Read the model definition and answer for the solid it produces. Units are mm, in the model's axes. A direction names the side the tool comes from. Coordinates: 2 decimals unless noted, no trailing zeros. Order: outer loops, then holes, each group sorted by start corner. A loop starts at its lowest first (then second) coordinate and runs counter-clockwise, first axis right, second up. Notation, with made-up numbers: M 63,69 L 106,69 A21 ccw 106,104 Z; hole C 9,69 d8. An arc over 180 degrees is marked long. One line per question, with ' | ' between items. Start each with the question number.
1) Consider probe 1 along X at (y, z) = (18.7, 40); probe 2 along Z at (x, y) = (-51.5, -15); probe 3 along Y at (x, z) = (65, 32). Determine where each line is inside the solid, lowest interval first.
2) Find section D-D, the plane z = 26. Write down the section's boundary in (x, y).
3) Find section A-A, the plane y = 0. Write down the section's boundary in (x, z), plus the area to 3 significant figures.
4) Given P1, Ø17.5, axis at x = -3.5, y = 2.5, coming from the +Z side; P2, Ø5, axis at y = 0.5, z = 6.5, coming from the -X side; P3, Ø5, axis at x = 53, z = 11, coming from the -Y side, each flat-ended and moving along its own axis, determine where each tip first touches the part or whether it passes through.
5) Find section C-C, the plane x = 50. Write down the section's boundary in (y, z), plus the area to 3 significant figures.
6) A tool of negligible diameter and unlimited length cuts with its end or side. For faces 5 (the face through (-1, 20, 28)), 6 (the face through (-1, -2, 2)), from which of +Z, -Z, +X, -X, +Y, -Y can it reach the whole face along a straight path? Write none if from no direction.
7) Find section B-B, the plane x = -4. Write down the section's boundary in (y, z).
8) The mould has two halves that part along Z. Classify faces 1 (the face through (-1.05, 18.645, 1.428)), 2 (the face through (-1, 18, 27)), 3 (the face through (-54, 19, 37)), 4 (the face through (46, 19, 37)): +Z half, -Z half, draft (parallel to the pull), parting line (faces both ways), or undercut.
Autodesk Inventor part; units mm, degrees
ref_plane "YZ Plane" through (0, 0, 0) normal (1, 0, 0) x (0, 1, 0)
ref_plane "XZ Plane" through (0, 0, 0) normal (0, 1, 0) x (-1, 0, 0)
ref_plane "XY Plane" through (0, 0, 0) normal (0, 0, 1) x (1, 0, 0)
sketch "Sketch1" plane through (0, 0, 0) normal (0, 0, 1) x (1, 0, 0)
  line L0 (-75, -20) -> (75, -20)
  line L1 (75, -20) -> (75, 20)
  line L2 (75, 20) -> (-75, 20)
  line L3 (-75, 20) -> (-75, -20)
  line L4 (-75, -20) -> (75, 20) construction
  line L5 (75, -20) -> (-75, 20) construction
  circle A0 centre (-48, 0) radius 9.5
  circle A1 centre (48, 0) radius 9.5
  line L6 (0, 20) -> (0, -20) construction
  point P0 (0, 0)
  point P1 (0, 0)
  dimension "d0" = 150
  dimension "d1" = 40
  dimension "d6" = 19
  dimension "d7" = 96
extrude "Plate1" add sketch "Sketch1" along normal blind 2
sketch "Sketch3" plane through (-75, 18, 0) normal (0, 1, 0) x (-1, 0, 0)
  line L0 (-150, 0) -> (0, 0)
  line L1 (0, 0) -> (0, 50)
  line L2 (0, 50) -> (-150, 50)
  line L3 (-150, 50) -> (-150, 0)
edge flange "Flange1" height 50 angle 90 thickness 2 bend radius 2.75 thickness toward (0, 1, 0) relief round relief width 2 relief depth 1 edges at (0, 20, 2) wall of the first edge with corners at (75, 18, 0) (-75, 18, 0) (-75, 18, 50) (75, 18, 50)
bend "Bend1"
corner "Corner1"
sketch "Sketch4" plane through (-75, 20, 50) normal (0, 1, 0) x (1, 0, 0)
  circle A0 centre (25, 10) radius 5
  circle A1 centre (125, 10) radius 5
  line L0 (150, 0) -> (0, 0) construction
  line L1 (75, 0) -> (75, 50) construction
  line L2 (150, 48) -> (0, 48) construction
  dimension "d18" = 10
  dimension "d19" = 10
  dimension "d20" = 100
extrude "Cut1" cut sketch "Sketch4" against normal blind 2
fillet "Corner Round1" radius 10 4 edges at (75, 19, 50) (-75, -20, 1) (-75, 19, 50) (75, -20, 1)
equation "\"d21\" = Thickness"
equation "\"d2\" = Thickness"
equation "\"d8\" = BendReliefWidth"
equation "\"d9\" = BendReliefDepth"
equation "\"d10\" = MinimumRemnant"
equation "\"d11\" = TransitionRadius"
equation "\"d14\" = BendRadius"
equation "\"d15\" = CornerReliefSize"
equation "\"d16\" = GapSize"
equation "\"d17\" = JacobiRadiusSize"
equation "\"BendReliefWidth\" = Thickness"
equation "\"BendReliefDepth\" = 0.5 * Thickness"
equation "\"CornerReliefSize\" = 4 * Thickness"
equation "\"MinimumRemnant\" = 2 * Thickness"
equation "\"TransitionRadius\" = BendRadius"
equation "\"JacobiRadiusSize\" = BendRadius"
equation "\"GapSize\" = Thickness"
properties part number "Goat_roller_supp" material "Stainless Steel"
Report:
1) probe 1: x = -75 to -55, -45 to 45, 55 to 75 | probe 2: z = 0 to 2 | probe 3: y = 18 to 20
2) outline: M -75,18 L 75,18 L 75,20 L -75,20 Z
3) outline: M -75,0 L -57.5,0 L -57.5,2 L -75,2 Z; M -38.5,0 L 38.5,0 L 38.5,2 L -38.5,2 Z; M 57.5,0 L 75,0 L 75,2 L 57.5,2 Z | area: 224 mm^2
4) P1: stops at z = 2 | P2: passes through | P3: stops at y = 18
5) outline: M -20,0 L -9.29,0 L -9.29,2 L -20,2 Z; M 9.29,0 L 15.25,0 A4.75 ccw 20,4.75 L 20,35 L 18,35 L 18,4.75 A2.75 cw 15.25,2 L 9.29,2 Z; M 18,45 L 20,45 L 20,50 L 18,50 Z | area: 116 mm^2
6) face 5: +Z, -Z, +X, -X, +Y | face 6: +Z, +X, -X, -Y
7) outline: M -20,0 L 15.25,0 A4.75 ccw 20,4.75 L 20,50 L 18,50 L 18,4.75 A2.75 cw 15.25,2 L -20,2 Z
8) face 1: -Z half | face 2: draft | face 3: undercut | face 4: undercut
